Part model, mm, in its own coordinate system. Face numbers are marked on the shaded views. A direction names the side the tool comes from. Round coordinates to 2 decimals unless told otherwise and drop trailing zeros. Write each loop counter-clockwise with the first axis right and the second up, starting at its lowest first coordinate (ties: lowest second). Pieces come first, ordered by that corner, then holes. Notation, with made-up numbers: M 69,43 L 98,43 A32 ccw 98,70 Z; hole C 3,-23 d4. An arc over 180 degrees is marked long. Use one line per item in the form item = value. Start each with the question number.
Item 1: Which spindle directions (+Z, -Z, +X, -X, +Y, -Y) get a long thin tool onto all of the face, cutting with end or side? Do the marked faces 3, 4 and 5. Say none if no direction does.
Item 2: Cut at C-C, the plane z = -9. Give the cut face in (x, y), then the cut area to 3 significant figures.
Item 3: Flat gauge pins, fed straight in: pin 1 Ø4 at (x, z) = (3, 0) entering from +Y; pin 2 Ø2 at (x, y) = (6, -4.5) entering from +Z; pin 3 Ø4 at (y, z) = (6.5, 1.5) entering from -X; pin 4 Ø10 at (x, y) = (-6, 5) entering from +Z. Where does each tip first touch, or does it go through?
Item 4: Cut at A-A, the plane y = 0. Give the cut face in (x, z), then the cut area to 3 significant figures.
Item 5: Probe L1, parallel to Z at x = 7, y = 0; L2, parallel to X at y = -11.5, z = 1; L3, parallel to Y at x = -1, z = 18.5. List the from-to ranges inside material, lowest first.
Item 6: Cut at D-D, the plane y = -8. Give the cut face in (x, z), then the cut area to 3 significant figures.
Item 7: Mould opens along Y. For the marked faces 1 and 2 say: +Y half, -Y half, draft (parallel to the pull), parting line (faces both ways), or undercut.
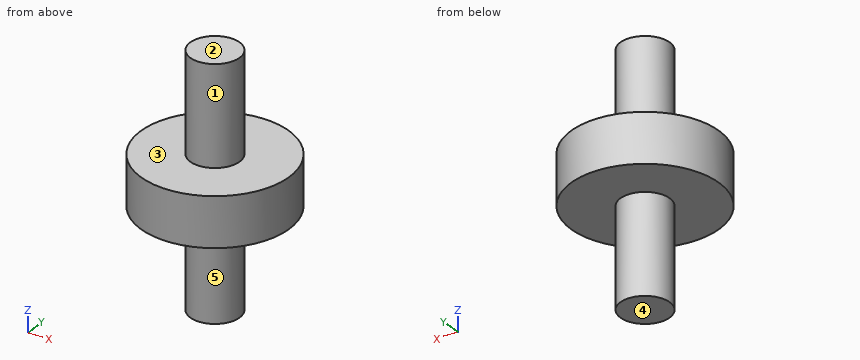
from build123d import *

# Parameters (mm, degrees)
SKETCH1_R                = 15
BOSS_EXTRUDE1_DEPTH      = 10
BOSS_EXTRUDE2_DEPTH      = 30
BOSS_EXTRUDE2_DEPTH_BACK = 20
SKETCH2_R                = 5


with BuildPart() as part:
    # Sketch1 → Boss-Extrude1 (new body)
    with BuildSketch(Plane.XY):
        Circle(SKETCH1_R)
    extrude(amount=BOSS_EXTRUDE1_DEPTH)

    # Sketch2 → Boss-Extrude2 (add, two sides: drawn at the far end of the back side and taken through both)
    with BuildSketch(Plane.XY.offset(-BOSS_EXTRUDE2_DEPTH_BACK)):
        Circle(SKETCH2_R)
    extrude(amount=BOSS_EXTRUDE2_DEPTH + BOSS_EXTRUDE2_DEPTH_BACK)


solid = part.part
Model answer:
q1.face_3 = +Z
q1.face_4 = -Z, +X, -X, +Y, -Y
q1.face_5 = -Z
q2.outline = C 0,0 d10
q2.area = 78.5 mm²
q3.pin_1 = 14.97
q3.pin_2 = 10
q3.pin_3 = -14.31
q3.pin_4 = 30
q4.outline = M -15,0 L -5,0 L -5,-20 L 5,-20 L 5,0 L 15,0 L 15,10 L 5,10 L 5,30 L -5,30 L -5,10 L -15,10 Z
q4.area = 700 mm²
q5.L1 = 0 to 10
q5.L2 = -9.63 to 9.63
q5.L3 = -4.9 to 4.9
q6.outline = M -12.69,0 L 12.69,0 L 12.69,10 L -12.69,10 Z
q6.area = 254 mm²
q7.face_1 = parting line
q7.face_2 = draft
